Geometry: see drawing. Coordinates: mm, zero at the bounding-box minimum. Round coordinates to 2 decimals unless told otherwise and drop trailing zeros. Order: outer loops, then holes, each group sorted by start corner. A loop starts at its lowest first (then second) coordinate and runs counter-clockwise, first axis right, second up. Notation, with made-up numbers: (-12.5, 70.5) -> (21.5, 70.5) arc R21 cw to (21.5, 95.5) -> close; hole circle Ø11 at (84.25, -34.75). An arc over 180 degrees is marked (long way). Answer as CSV lines item,"result". Start each with the question number.
(1) Section query A-A (z = 15). Output: boundary loops of the cut face in (x, y), plus the area to 3 significant figures.
(2) Contact query for a flat-ended pin moving along its axis: P1, Ø8.5, axis at x = 100, z = 15, coming from the -Y side. Output: stop coordinate, or through.
(3) Line query: line 1 along X through (y, z) = (7.75, 15); line 2 along Z through (x, y) = (1040, 4.5); line 3 along X through (y, z) = (3, 19.75). Output: solid intervals per line, ascending. Write a range as from..to.
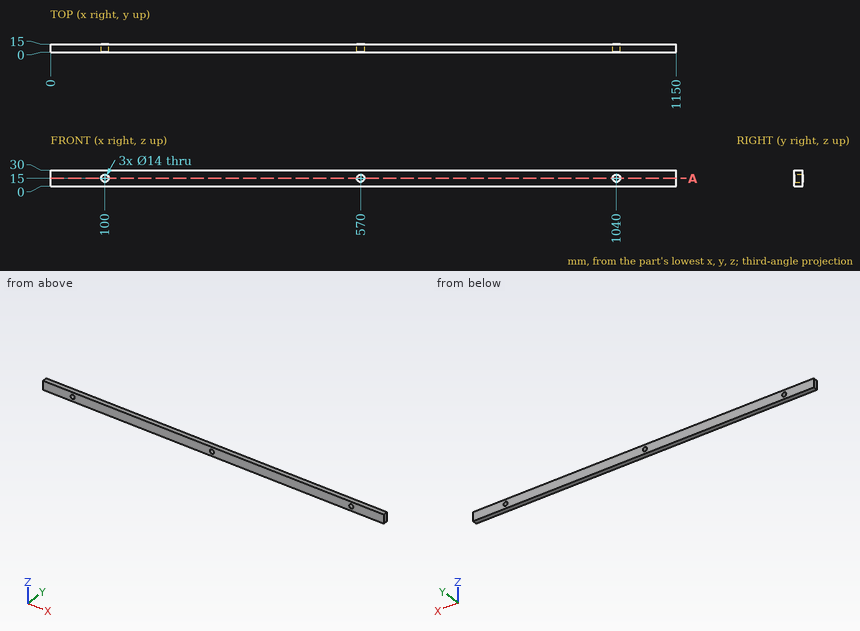
Answer block:
1,outline,"(0, 0) -> (93, 0) -> (93, 15) -> (0, 15) -> close; (107, 0) -> (563, 0) -> (563, 15) -> (107, 15) -> close; (577, 0) -> (1033, 0) -> (1033, 15) -> (577, 15) -> close; (1047, 0) -> (1150, 0) -> (1150, 15) -> (1047, 15) -> close"
1,area,"16,600 mm2"
2,P1,"through"
3,line 1,"0..93, 107..563, 577..1033, 1047..1150"
3,line 2,"0..8, 22..30"
3,line 3,"0..94.86, 105.14..564.86, 575.14..1034.86, 1045.14..1150"
